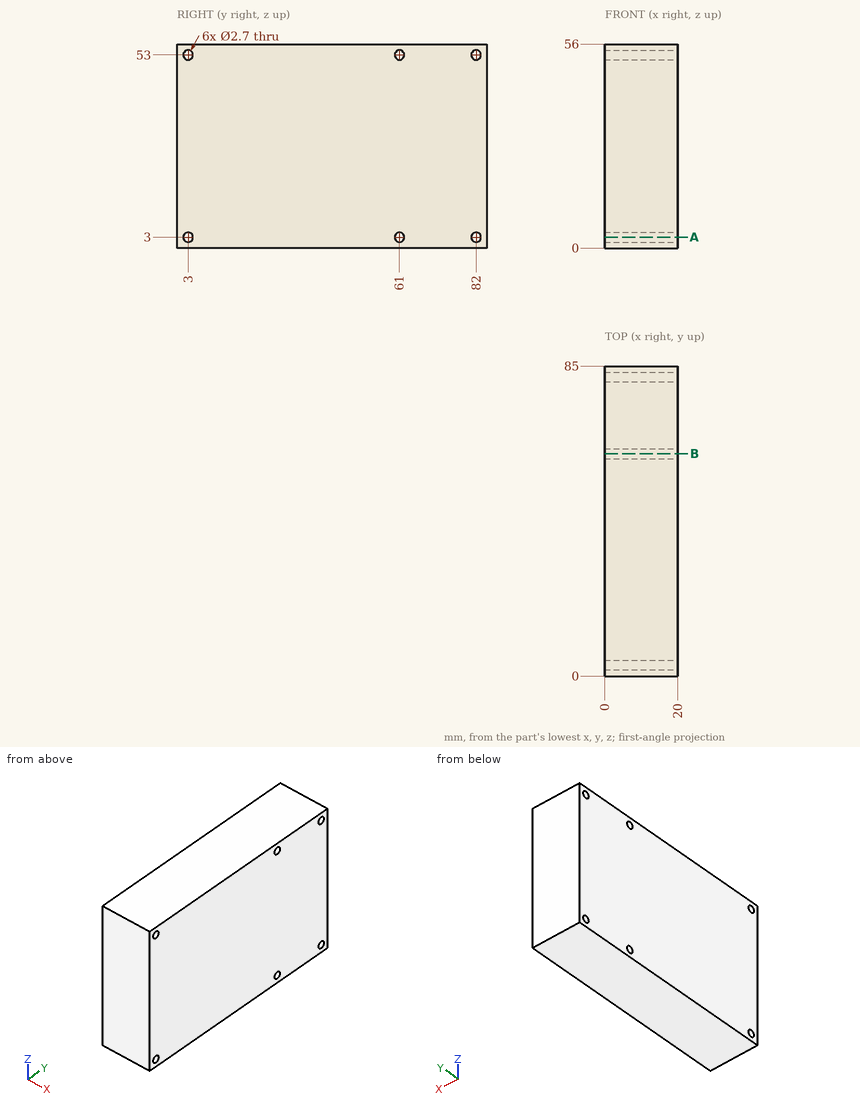
Drawing for the job (mm, zero at the part's lowest x, y, z). Round coordinates to 2 decimals unless told otherwise and drop trailing zeros. Write each loop counter-clockwise with the first axis right and the second up, starting at its lowest first coordinate (ties: lowest second). Pieces come first, ordered by that corner, then holes.
Item 1: Band-saw the part on A-A on z = 3. Write the cut outline in (x, y), then the cut area to 3 significant figures.
Filled in:
outline: (0, 0) - (20, 0) - (20, 1.65) - (0, 1.65) - close; (0, 4.35) - (20, 4.35) - (20, 59.65) - (0, 59.65) - close; (0, 62.35) - (20, 62.35) - (20, 80.65) - (0, 80.65) - close; (0, 83.35) - (20, 83.35) - (20, 85) - (0, 85) - close
area: 1,540 mm2
Item 2: Band-saw the part on B-B on y = 61. Write the cut outline in (x, z).
Filled in:
outline: (0, 0) - (20, 0) - (20, 1.65) - (0, 1.65) - close; (0, 4.35) - (20, 4.35) - (20, 51.65) - (0, 51.65) - close; (0, 54.35) - (20, 54.35) - (20, 56) - (0, 56) - close
Item 3: Drill centre lines: L1, parallel to Y at x = 9, z = 3; L2, parallel to Z at x = 7.75, y = 82; L3, parallel to Z at x = 14.75, y = 62. Where is each one in solid material? Low to high.
Filled in:
L1: y = 0 to 1.65, 4.35 to 59.65, 62.35 to 80.65, 83.35 to 85
L2: z = 0 to 1.65, 4.35 to 51.65, 54.35 to 56
L3: z = 0 to 2.09, 3.91 to 52.09, 53.91 to 56
